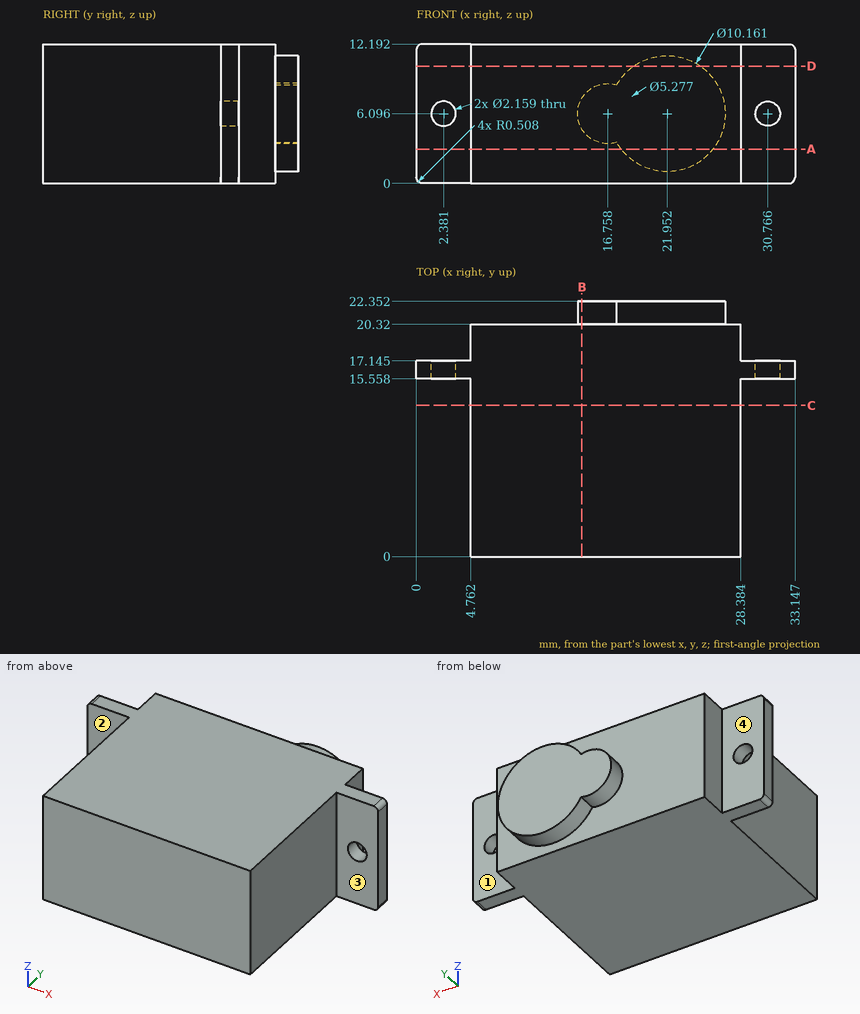
Print and shaded views of the part. All mm, measured from the part's lowest x, y and z. A direction names the side the tool comes from. Coordinates: 2 decimals unless noted, no trailing zeros. Loops run counter-clockwise (first coordinate to the right, second up) from the corner with the lowest first, then second, coordinate; pieces in that order, holes last. Notation, with made-up numbers: (6, -24.5) -> (64, -24.5) arc R20 ccw to (64, 10.5) -> close; hole circle Ø6 at (-30.75, 55). An arc over 180 degrees is marked (long way). Use one line per item in the form item = value. Start each with the question number.
(1) Cut at C-C on y = 13.25. Give the cut face in (x, z) (1 decimal), and give its area (3 significant figures).
(2) Cut at D-D on z = 10.25. Give the cut face in (x, y) (1 decimal).
(3) Flat gauge pins, fed straight in: pin 1 (1.5 mm diameter, centred on x = 7, z = 3, fed in from +Y); pin 2 (2.5 mm diameter, centred on x = 3, z = 8, fed in from -Y); pin 3 (4 mm diameter, centred on x = 31, z = 4.5, fed in from +Y) (1 decimal); pin 4 (1.7 mm diameter, centred on x = 2.38, z = 6.1, fed in from +Y). Where does each tip first touch, or does it go through?
(4) Probe probe 1 along X at (y, z) = (14.25, 9.5) (1 decimal); probe 2 along Y at (x, z) = (27, 10.25); probe 3 along Y at (x, z) = (30, 10) (1 decimal). List the from-to ranges inside material, lowest first. Write a range as from..to.
(5) Cut at A-A on z = 3. Give the cut face in (x, y) (1 decimal).
(6) Tool access for the marked faces 1, 2, 3 and 4: list every direction of +Z, -Z, +X, -X, +Y, -Y with a clear straight run to the whole face (end or side of a thin tool).
(7) Cut at B-B on x = 14.5. Give the cut face in (y, z), and give its area (3 significant figures).
Values:
q1.outline = (4.8, 0) -> (28.4, 0) -> (28.4, 12.2) -> (4.8, 12.2) -> close
q1.area = 288 mm2
q2.outline = (0, 15.6) -> (4.8, 15.6) -> (4.8, 0) -> (28.4, 0) -> (28.4, 15.6) -> (33.1, 15.6) -> (33.1, 17.1) -> (28.4, 17.1) -> (28.4, 20.3) -> (24.9, 20.3) -> (24.9, 22.4) -> (19, 22.4) -> (19, 20.3) -> (4.8, 20.3) -> (4.8, 17.1) -> (0, 17.1) -> close
q3.pin_1 = 20.32
q3.pin_2 = 15.56
q3.pin_3 = 17.1
q3.pin_4 = through
q4.probe_1 = 4.8..28.4
q4.probe_2 = 0..20.32
q4.probe_3 = 15.6..17.1
q5.outline = (0, 15.6) -> (4.8, 15.6) -> (4.8, 0) -> (28.4, 0) -> (28.4, 15.6) -> (33.1, 15.6) -> (33.1, 17.1) -> (28.4, 17.1) -> (28.4, 20.3) -> (26, 20.3) -> (26, 22.4) -> (17.9, 22.4) -> (17.9, 20.3) -> (4.8, 20.3) -> (4.8, 17.1) -> (0, 17.1) -> close
q6.face_1 = +Z, -Z, +X, +Y
q6.face_2 = +Z, -Z, -X, -Y
q6.face_3 = +Z, -Z, +X, -Y
q6.face_4 = +Z, -Z, -X, +Y
q7.outline = (0, 0) -> (20.32, 0) -> (20.32, 4.73) -> (22.35, 4.73) -> (22.35, 7.46) -> (20.32, 7.46) -> (20.32, 12.19) -> (0, 12.19) -> close
q7.area = 253 mm2
